```python
from build123d import *

# Parameters (mm, degrees)
SKETCH2_R           = 1.6
BOSS_EXTRUDE2_DEPTH = 4
FILLET1_R           = 2
FILLET2_R           = 2
FILLET3_R           = 2
FILLET4_R           = 2


with BuildPart() as part:
    # Sketch2 → Boss-Extrude2 (new body)
    with BuildSketch(Plane(origin=(0, 0, 0), x_dir=(1, 0, 0), z_dir=(0, 1, 0))):
        Polygon((0, 28.53), (0, 0), (120, 0), (120, 28.53), (100.17, 28.53), (100.17, 51.47), (120, 51.47), (120, 80), (0, 80), (0, 51.47), (19.83, 51.47), (19.83, 28.53), align=None)
        with Locations((3, 3)):
            Circle(SKETCH2_R, mode=Mode.SUBTRACT)
        with Locations((23.43, 35)):
            Circle(SKETCH2_R, mode=Mode.SUBTRACT)
        with Locations((60, 3)):
            Circle(SKETCH2_R, mode=Mode.SUBTRACT)
        with Locations((117, 3)):
            Circle(SKETCH2_R, mode=Mode.SUBTRACT)
        with Locations((96.57, 35)):
            Circle(SKETCH2_R, mode=Mode.SUBTRACT)
        with Locations((23.43, 45)):
            Circle(SKETCH2_R, mode=Mode.SUBTRACT)
        with Locations((3, 77)):
            Circle(SKETCH2_R, mode=Mode.SUBTRACT)
        with Locations((96.57, 45)):
            Circle(SKETCH2_R, mode=Mode.SUBTRACT)
        with Locations((60, 77)):
            Circle(SKETCH2_R, mode=Mode.SUBTRACT)
        with Locations((117, 77)):
            Circle(SKETCH2_R, mode=Mode.SUBTRACT)
    extrude(amount=BOSS_EXTRUDE2_DEPTH)

    # Fillet1
    fillet1_edges = [part.edges().sort_by_distance(p)[0] for p in [
        (0, 2, -80),
    ]]
    fillet(fillet1_edges, radius=FILLET1_R)

    # Fillet2
    fillet2_edges = [part.edges().sort_by_distance(p)[0] for p in [
        (120, 2, -80),
    ]]
    fillet(fillet2_edges, radius=FILLET2_R)

    # Fillet3
    fillet3_edges = [part.edges().sort_by_distance(p)[0] for p in [
        (120, 2, 0),
    ]]
    fillet(fillet3_edges, radius=FILLET3_R)

    # Fillet4
    fillet4_edges = [part.edges().sort_by_distance(p)[0] for p in [
        (0, 2, 0),
    ]]
    fillet(fillet4_edges, radius=FILLET4_R)


solid = part.part
```
Geometry check sheet. Reference: the model listing, model coordinates, mm. A direction names the side the tool comes from. Give positions to 0.01 mm unless a question says otherwise; leave off trailing zeros. Order: outer loops, then holes, each group sorted by start corner. A loop starts at its lowest first (then second) coordinate and runs counter-clockwise, first axis right, second up. Notation, with made-up numbers: (-26.5, 52) - (-3.5, 52) arc R9 ccw to (-3.5, 62) - close; hole circle Ø10 at (28, 55.25). An arc over 180 degrees is marked (long way). Answer in a Markdown table with one row per item. Add a question column.
Q1. Cross-section at C-C, the plane z = -45. Enter the section's corners in (x, y), then the cut area to 3 significant figures.
Q2. Tool access check on faces 1 (the flat face through (110, 2, -28.53)), 2 (the flat face through (19.83, 2, -40)), 3 (the cylindrical face through (118.526, 1.972, -77.481)). Record the directions out of +Z, -Z, +X, -X, +Y, -Y that give a thin tool (end or side, any length) a straight path to the whole face; none if there is none.
Q3. Mould release check, pull along X, two halves, no side actions. Record for faces 4 (the flat face through (110, 2, -51.47)), 5 (the flat face through (0, 2, -15)), 6 (the cylindrical face through (118.526, 1.972, -3.481)): pulls with the +X half, pulls with the -X half, needs draft (parallel to the pull), parting line crosses it, or undercut.
Q4. Cross-section at B-B, the plane y = 2.9. Count the separate pieces of the cut face and the enclosed holes in it, then the cut area to 3 significant figures.
Q5. Cross-section at A-A, the plane x = 60. Enter the section's corners in (y, z), then the cut area to 3 significant figures.
Q6. Gauge pin test, flat ends, axial feed: pin 1 (4 mm diameter, centred on x = 23.43, z = -35, fed in from -Y); pin 2 (3 mm diameter, centred on x = 60, z = -77, fed in from +Y); pin 3 (1 mm diameter, centred on y = 0.5, z = -32, fed in from -X). Record the tip position at first contact, or that the pin passes through.
Q7. Cross-section at D-D, the plane x = 107.5. Enter the section's corners in (y, z), then the cut area to 3 significant figures.
Q8. Material ranges on probe 1 along Z at (x, y) = (60, 2.6); probe 2 along X at (y, z) = (1.85, -35); probe 3 along X at (y, z) = (1.6, -3), recorded low to high. Write a range as from..to.
Check values:
| question | item | result |
|---|---|---|
| 1 | outline | (19.83, 0) - (21.83, 0) - (21.83, 4) - (19.83, 4) - close; (25.03, 0) - (94.97, 0) - (94.97, 4) - (25.03, 4) - close; (98.17, 0) - (100.17, 0) - (100.17, 4) - (98.17, 4) - close |
| 1 | area | 296 mm^2 |
| 2 | face 1 | +X, +Y, -Y |
| 2 | face 2 | -X, +Y, -Y |
| 2 | face 3 | +Y, -Y |
| 3 | face 4 | needs draft |
| 3 | face 5 | pulls with the -X half |
| 3 | face 6 | undercut |
| 4 | separate pieces | 1 |
| 4 | enclosed holes | 10 |
| 4 | area | 8,610 mm^2 |
| 5 | outline | (0, -80) - (4, -80) - (4, -78.6) - (0, -78.6) - close; (0, -75.4) - (4, -75.4) - (4, -4.6) - (0, -4.6) - close; (0, -1.4) - (4, -1.4) - (4, 0) - (0, 0) - close |
| 5 | area | 294 mm^2 |
| 6 | pin 1 | stops at y = 0 |
| 6 | pin 2 | passes through |
| 6 | pin 3 | stops at x = 19.83 |
| 7 | outline | (0, -80) - (4, -80) - (4, -51.47) - (0, -51.47) - close; (0, -28.53) - (4, -28.53) - (4, 0) - (0, 0) - close |
| 7 | area | 228 mm^2 |
| 8 | probe 1 | z = -80..-78.6, -75.4..-4.6, -1.4..0 |
| 8 | probe 2 | x = 19.83..21.83, 25.03..94.97, 98.17..100.17 |
| 8 | probe 3 | x = 0..1.4, 4.6..58.4, 61.6..115.4, 118.6..120 |
